Geometry: see drawing. Coordinates: mm, zero at the bounding-box minimum. Coordinates: 2 decimals unless noted, no trailing zeros. Write each loop counter-clockwise with the first axis right and the second up, starting at its lowest first coordinate (ties: lowest second). Pieces come first, ordered by that corner, then holes.
1) Section query B-B (y = 10). Output: boundary loops of the cut face in (x, z), then the cut area to 4 significant figures.
2) Line query: L1, parallel to Y at x = 5.5, z = 3; L2, parallel to X at y = 45, z = 12.25; L3, parallel to Y at x = 6.75, z = 10. Output: solid intervals per line, ascending.
3) Section query A-A (z = 7.5). Output: boundary loops of the cut face in (x, y), then the cut area to 3 significant figures.
4) Section query C-C (x = 4.75). Output: boundary loops of the cut face in (y, z).
5) Section query D-D (z = 3.75). Output: boundary loops of the cut face in (x, y), then the cut area to 3 significant figures.
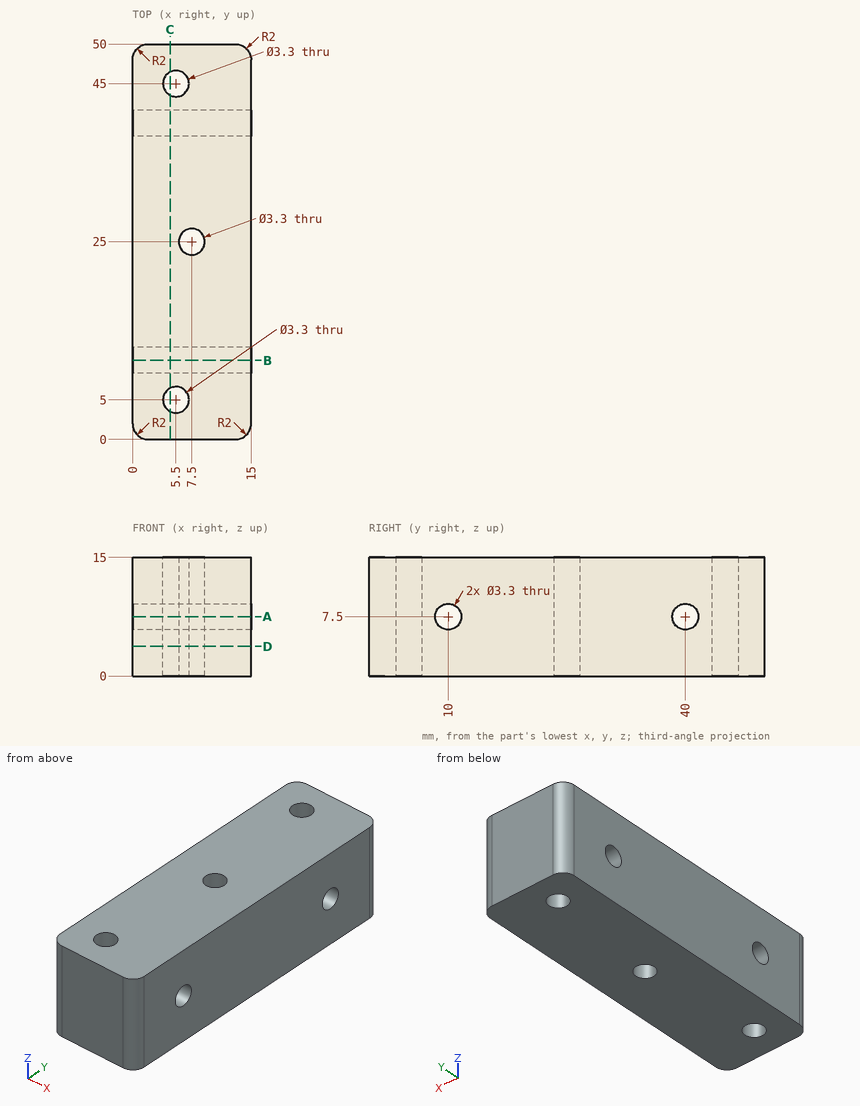
Answer:
1. outline: (0, 0) - (15, 0) - (15, 5.85) - (0, 5.85) - close; (0, 9.15) - (15, 9.15) - (15, 15) - (0, 15) - close
1. area: 175.5 mm2
2. L1: y = 0 to 3.35, 6.65 to 43.35, 46.65 to 50
2. L2: x = 0 to 3.85, 7.15 to 15
2. L3: y = 0 to 3.92, 6.08 to 23.53, 26.47 to 43.92, 46.08 to 50
3. outline: (0, 2) arc R2 ccw to (2, 0) - (13, 0) arc R2 ccw to (15, 2) - (15, 8.35) - (0, 8.35) - close; (0, 11.65) - (15, 11.65) - (15, 38.35) - (0, 38.35) - close; (0, 41.65) - (15, 41.65) - (15, 48) arc R2 ccw to (13, 50) - (2, 50) arc R2 ccw to (0, 48) - close; hole circle Ø3.3 at (5.5, 5); hole circle Ø3.3 at (5.5, 45); hole circle Ø3.3 at (7.5, 25)
3. area: 622 mm2
4. outline: (0, 0) - (3.53, 0) - (3.53, 15) - (0, 15) - close; (6.47, 0) - (43.53, 0) - (43.53, 15) - (6.47, 15) - close; (46.47, 0) - (50, 0) - (50, 15) - (46.47, 15) - close; hole circle Ø3.3 at (10, 7.5); hole circle Ø3.3 at (40, 7.5)
5. outline: (0, 2) arc R2 ccw to (2, 0) - (13, 0) arc R2 ccw to (15, 2) - (15, 48) arc R2 ccw to (13, 50) - (2, 50) arc R2 ccw to (0, 48) - close; hole circle Ø3.3 at (5.5, 5); hole circle Ø3.3 at (5.5, 45); hole circle Ø3.3 at (7.5, 25)
5. area: 721 mm2
